Here's how the part is built. I have some questions about the finished solid (model axes, mm). A direction names the side the tool comes from. Round coordinates to 2 decimals unless told otherwise and drop trailing zeros. Loops run counter-clockwise (first coordinate to the right, second up) from the corner with the lowest first, then second, coordinate; pieces in that order, holes last. Notation, with made-up numbers: (41, -24.75) -> (72, -24.75) arc R13 cw to (72, -2.75) -> close; hole circle Ø4 at (73.5, 8.25). An arc over 180 degrees is marked (long way). One line per item, written item: value. Start each with the question number.
```python
from build123d import *

# Parameters (mm, degrees)
SKETCH1_W           = 10
SKETCH1_H           = 6
BOSS_EXTRUDE1_DEPTH = 2.5
SKETCH2_W           = 12
SKETCH2_H           = 6
BOSS_EXTRUDE2_DEPTH = 1
FILLET1_R           = 1


with BuildPart() as part:
    # Sketch1 → Boss-Extrude1 (new body)
    with BuildSketch(Plane(origin=(0, 0, 0), x_dir=(1, 0, 0), z_dir=(0, 1, 0))):
        Rectangle(SKETCH1_W, SKETCH1_H)
    extrude(amount=BOSS_EXTRUDE1_DEPTH)

    # Sketch2 → Boss-Extrude2 (add)
    with BuildSketch(Plane.XZ):
        Rectangle(SKETCH2_W, SKETCH2_H)
    extrude(amount=BOSS_EXTRUDE2_DEPTH)

    # Fillet1
    fillet1_edges = [part.edges().sort_by_distance(p)[0] for p in [
        (6, -0.5, 3),
        (-6, -0.5, 3),
        (-5, 1.25, 3),
        (5, 1.25, 3),
        (6, -0.5, -3),
        (-6, -0.5, -3),
        (5, 1.25, -3),
        (-5, 1.25, -3),
    ]]
    fillet(fillet1_edges, radius=FILLET1_R)


solid = part.part
```
Q1. I want a section at B-B on y = 0.4. Please give me the cut outline in (x, z), plus the area to 3 significant figures.
Q2. If I drill on line 1 along X through (y, z) = (1.7, 1.95); line 2 along Y through (x, z) = (5, -2.35); line 3 along X through (y, z) = (-0.35, 2.6), over which ranges is the centre line in solid material (lowest first)?
Q3. Which directions (+Z, -Z, +X, -X, +Y, -Y) give clear straight access to the entire face, cutting with the end or side of a thin tool? Please do faces 1 (the cylindrical face through (-4.699, 1.268, -2.715)), 2 (the cylindrical face through (4.699, 1.268, -2.715)), 3 (the cylindrical face through (-4.699, 1.268, 2.715)).
Q4. I want a section at A-A on z = 1.5. Please give me the cut outline in (x, y), plus the area to 3 significant figures.
Q5. Will these pins go through, and if not, where does the flat tip stop? P1, Ø1, axis at y = 2, z = 2, coming from the +X side; P2, Ø0.8, axis at y = 1, z = 0.5, coming from the -X side.
Answers below:
1. outline: (-5, -2) arc R1 ccw to (-4, -3) -> (4, -3) arc R1 ccw to (5, -2) -> (5, 2) arc R1 ccw to (4, 3) -> (-4, 3) arc R1 ccw to (-5, 2) -> close
1. area: 59.1 mm^2
2. line 1: x = -5 to 5
2. line 2: y = -1 to 0
2. line 3: x = -5.8 to 5.8
3. face 1: -Z, -X, +Y
3. face 2: -Z, +X, +Y
3. face 3: +Z, -X, +Y
4. outline: (-6, -1) -> (6, -1) -> (6, 0) -> (5, 0) -> (5, 2.5) -> (-5, 2.5) -> (-5, 0) -> (-6, 0) -> close
4. area: 37.0 mm^2
5. P1: stops at x = 5
5. P2: stops at x = -5
